Autodesk Inventor part; units mm, degrees
ref_plane "YZ Plane" through (0, 0, 0) normal (1, 0, 0) x (0, 1, 0)
ref_plane "XZ Plane" through (0, 0, 0) normal (0, 1, 0) x (-1, 0, 0)
ref_plane "XY Plane" through (0, 0, 0) normal (0, 0, 1) x (1, 0, 0)
sketch "Sketch1" plane through (0, 0, 0) normal (0, 1, 0) x (-1, 0, 0)
  line L0 (0, 0) -> (2150, 0)
  line L1 (2150, 0) -> (2150, 600)
  line L2 (2150, 600) -> (600, 600)
  line L3 (600, 600) -> (600, 1550)
  line L4 (600, 1550) -> (0, 1550)
  line L5 (0, 1550) -> (0, 0)
  dimension "d0" = 2150
  dimension "d1" = 600
  dimension "d2" = 1550
extrude "Extrusion1" add sketch "Sketch1" along normal blind 20
sketch "Sketch2" plane through (0, 20, 0) normal (0, 1, 0) x (1, 0, 0)
  line L0 (-725, -500) -> (-1375, -500)
  line L1 (-1375, -500) -> (-1375, -100)
  line L2 (-1375, -100) -> (-725, -100)
  line L3 (-725, -100) -> (-725, -500)
  line L4 (-725, -500) -> (-1375, -100) construction
  line L5 (-1375, -500) -> (-725, -100) construction
  line L6 (-2150, 0) -> (-2150, -600)
  line L7 (0, 0) -> (-2150, 0)
  line L8 (-500, -1350) -> (-100, -1350)
  line L9 (-100, -1350) -> (-100, -750)
  line L10 (-100, -750) -> (-500, -750)
  line L11 (-500, -750) -> (-500, -1350)
  line L12 (-500, -1350) -> (-100, -750) construction
  line L13 (-100, -1350) -> (-500, -750) construction
  line L14 (-600, -1550) -> (0, -1550)
  line L15 (0, -1550) -> (0, 0)
  point P0 (-1050, -300)
  point P1 (-300, -1050)
  dimension "d5" = 650
  dimension "d6" = 400
  dimension "d8" = 300
  dimension "d9" = 400
  dimension "d10" = 600
  dimension "d12" = 300
  dimension "d16" = 1050
  dimension "d17" = 1050
extrude "Extrusion2" cut sketch "Sketch2" against normal through all
fillet "Fillet1" radius 20 8 edges at (-725, 10, 500) (-725, 10, 100) (-1375, 10, 100) (-1375, 10, 500) (-500, 10, 1350) (-100, 10, 1350) (-100, 10, 750) (-500, 10, 750)
properties part number "Top cucina"
The listing builds one solid part. Answer for the finished solid, in the listing's coordinates (mm). Coordinates: 2 decimals unless noted, no trailing zeros. Loops run counter-clockwise (first coordinate to the right, second up) from the corner with the lowest first, then second, coordinate; pieces in that order, holes last. Notation, with made-up numbers: (25.25, -31.5) -> (34.25, -31.5) arc R10 ccw to (34.25, -27.5) -> close; hole circle Ø4 at (-32.75, -30). An arc over 180 degrees is marked (long way). Use one line per item in the form item = value. Start each with the question number.
Item 1: A flat-ended cylindrical pin translates along its axis: pin 1 Ø1.5 at (x, y) = (-1714, 12.5) entering from +Z. Find the tip coordinate at first contact, or state that the pin passes through.
Item 2: The part is cut by section A-A on z = 1303. Determine the outline of the cut face in (x, y).
Item 3: The part is cut by section C-C on x = -1145.5. Determine the outline of the cut face in (y, z).
Item 4: The part is cut by section D-D on x = -1939.5. Determine the outline of the cut face in (y, z), then the cut area to 3 significant figures.
Item 5: The part is cut by section B-B on y = 11.5. Determine the outline of the cut face in (x, z), then the cut area to 3 significant figures.
Item 6: Consider L1, parallel to X at y = 18.25, z = 1142; L2, parallel to X at y = 14.75, z = 248; L3, parallel to Z at x = -469, y = 2.5. Determine where each line is inside the solid, lowest interval first. Write a range as [from, to].
Answer key:
q1.pin_1 = 600
q2.outline = (-600, 0) -> (-500, 0) -> (-500, 20) -> (-600, 20) -> close; (-100, 0) -> (0, 0) -> (0, 20) -> (-100, 20) -> close
q3.outline = (0, 0) -> (20, 0) -> (20, 100) -> (0, 100) -> close; (0, 500) -> (20, 500) -> (20, 600) -> (0, 600) -> close
q4.outline = (0, 0) -> (20, 0) -> (20, 600) -> (0, 600) -> close
q4.area = 12,000 mm2
q5.outline = (-2150, 0) -> (0, 0) -> (0, 1550) -> (-600, 1550) -> (-600, 600) -> (-2150, 600) -> close; hole (-1375, 120) arc R20 ccw to (-1355, 100) -> (-745, 100) arc R20 ccw to (-725, 120) -> (-725, 480) arc R20 ccw to (-745, 500) -> (-1355, 500) arc R20 ccw to (-1375, 480) -> close; hole (-500, 770) arc R20 ccw to (-480, 750) -> (-120, 750) arc R20 ccw to (-100, 770) -> (-100, 1330) arc R20 ccw to (-120, 1350) -> (-480, 1350) arc R20 ccw to (-500, 1330) -> close
q5.area = 1,360,000 mm2
q6.L1 = [-600, -500], [-100, 0]
q6.L2 = [-2150, -1375], [-725, 0]
q6.L3 = [0, 750], [1350, 1550]
